Check sheet for the drawn part. Datum: minimum x, y, z corner. Units: mm. Give positions to 0.01 mm unless a question says otherwise; leave off trailing zeros. Order: outer loops, then holes, each group sorted by start corner. A loop starts at its lowest first (then second) coordinate and runs counter-clockwise, first axis right, second up.
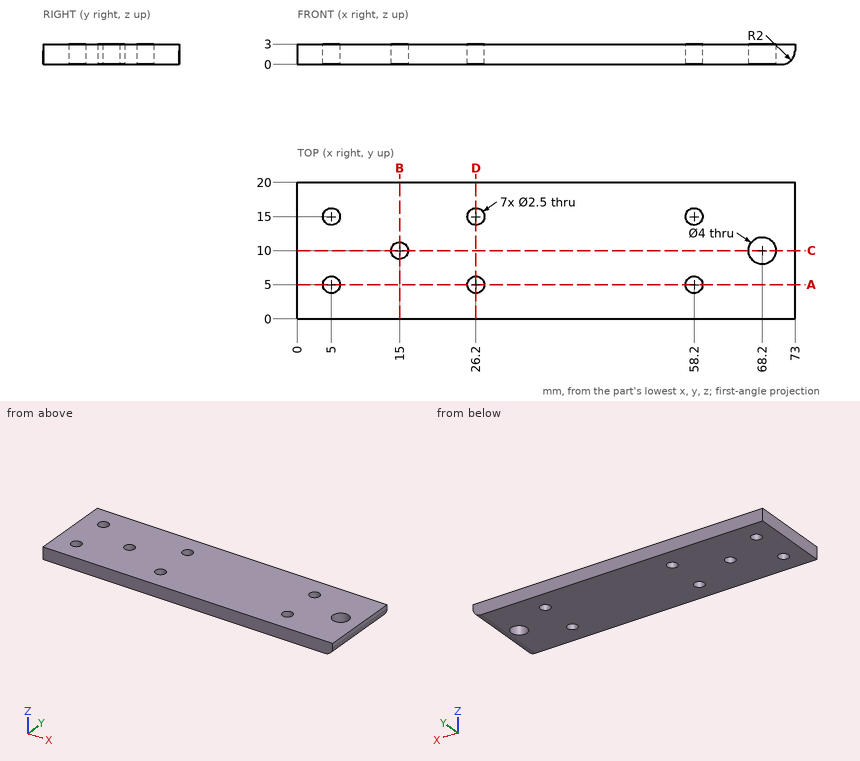
(1) Section check B-B, the plane x = 15. Enter the section's corners in (y, z).
Solved:
outline: (0, 0) - (8.75, 0) - (8.75, 3) - (0, 3) - close; (11.25, 0) - (20, 0) - (20, 3) - (11.25, 3) - close
(2) Go/stop test with a flat-tipped pin: pin 1 (3.5 mm diameter, centred on x = 68.2, y = 10, fed in from -Z). Record where the tip stops, or that it passes through.
Solved:
pin 1: passes through
(3) Section check A-A, the plane y = 5. Enter the section's corners in (x, z), then the cut area to 3 significant figures.
Solved:
outline: (0, 0) - (3.75, 0) - (3.75, 3) - (0, 3) - close; (6.25, 0) - (24.95, 0) - (24.95, 3) - (6.25, 3) - close; (27.45, 0) - (56.95, 0) - (56.95, 3) - (27.45, 3) - close; (59.45, 0) - (71, 0) arc R2 ccw to (73, 2) - (73, 3) - (59.45, 3) - close
area: 196 mm2
(4) Section check C-C, the plane y = 10. Enter the section's corners in (x, z), then the cut area to 3 significant figures.
Solved:
outline: (0, 0) - (13.75, 0) - (13.75, 3) - (0, 3) - close; (16.25, 0) - (66.2, 0) - (66.2, 3) - (16.25, 3) - close; (70.2, 0) - (71, 0) arc R2 ccw to (73, 2) - (73, 3) - (70.2, 3) - close
area: 199 mm2
(5) Section check D-D, the plane x = 26.2. Enter the section's corners in (y, z), then the cut area to 3 significant figures.
Solved:
outline: (0, 0) - (3.75, 0) - (3.75, 3) - (0, 3) - close; (6.25, 0) - (13.75, 0) - (13.75, 3) - (6.25, 3) - close; (16.25, 0) - (20, 0) - (20, 3) - (16.25, 3) - close
area: 45.0 mm2
(6) Scan lines: line 1 (Y direction, x = 26.2, z = 1); line 2 (X direction, y = 5.75, z = 1.45); line 3 (X direction, y = 6, z = 2.85). Record each from-to range of solid material in increasing order.
Solved:
line 1: y = 0 to 3.75, 6.25 to 13.75, 16.25 to 20
line 2: x = 0 to 4, 6 to 25.2, 27.2 to 57.2, 59.2 to 72.92
line 3: x = 0 to 4.25, 5.75 to 25.45, 26.95 to 57.45, 58.95 to 73
